Can you work these out from the model? Positions are in its coordinate system, mm. Face numbers are marked on the shaded views. A direction names the side the tool comes from. Coordinates: 2 decimals unless noted, no trailing zeros. Write each loop counter-clockwise with the first axis right and the second up, starting at its lowest first coordinate (ties: lowest second). Pieces come first, ordered by that corner, then holes. Notation, with made-up numbers: (-17.5, 48.5) - (16.5, 48.5) arc R6 ccw to (16.5, 53.5) - close; hole circle Ø11 at (38, 33.5). An arc over 180 degrees is marked (long way). One line per question, with ' | ' between items. Start each with the question number.
from build123d import *

# Parameters (mm, degrees)
SKETCH2_R           = 76.2
BOSS_EXTRUDE2_DEPTH = 50.8
FILLET1_R           = 25.4
SKETCH3_W           = 25.4
SKETCH3_H           = 25.4
BOSS_EXTRUDE3_DEPTH = 25.4
CUT_EXTRUDE2_REACH  = 154.532
SKETCH5_R           = 6.35
CUT_EXTRUDE3_REACH  = 154.532
SKETCH6_R           = 6.35


with BuildPart() as part:
    # Sketch2 → Boss-Extrude2 (new body)
    with BuildSketch(Plane(origin=(0, 0, 0), x_dir=(1, 0, 0), z_dir=(0, 1, 0))):
        with Locations(Location((0, 0, 0), (0, 0, 270))):
            Circle(SKETCH2_R)
    extrude(amount=BOSS_EXTRUDE2_DEPTH)

    # Fillet1
    fillet1_edges = [part.edges().sort_by_distance(p)[0] for p in [
        (0, 50.8, -76.2),
    ]]
    fillet(fillet1_edges, radius=FILLET1_R)

    # Sketch3 → Boss-Extrude3 (add)
    with BuildSketch(Plane(origin=(0, 50.8, 0), x_dir=(1, 0, 0), z_dir=(0, 1, 0))):
        with Locations((-19.05, 19.05)):
            Rectangle(SKETCH3_W, SKETCH3_H)
        with Locations((19.05, 19.05)):
            Rectangle(SKETCH3_W, SKETCH3_H)
        with Locations((-19.05, -19.05)):
            Rectangle(SKETCH3_W, SKETCH3_H)
        with Locations((19.05, -19.05)):
            Rectangle(SKETCH3_W, SKETCH3_H)
    extrude(amount=BOSS_EXTRUDE3_DEPTH)

    # Cut-Extrude2: up to this face of the body (flat: up to its plane)
    cut_extrude2_end = Plane(part.part.faces().sort_by_distance((31.75, 63.5, -19.05))[0])
    # Sketch5 → Cut-Extrude2 (cut, up to the picked face)
    with BuildSketch(Plane.ZY.offset(31.75), mode=Mode.PRIVATE) as cut_extrude2_sk1:
        with Locations((-19.05, 63.5)):
            Circle(SKETCH5_R)
    cut_extrude2_tool1 = split(extrude(cut_extrude2_sk1.sketch, amount=-CUT_EXTRUDE2_REACH, mode=Mode.PRIVATE), bisect_by=cut_extrude2_end, keep=Keep.BOTH, mode=Mode.PRIVATE)
    add(cut_extrude2_tool1.solids().sort_by(Axis((-31.75, 63.5, -19.05), (1, 0, 0)))[0], mode=Mode.SUBTRACT)

    # Cut-Extrude3: up to this face of the body (flat: up to its plane)
    cut_extrude3_end = Plane(part.part.faces().sort_by_distance((31.75, 63.5, 19.05))[0])
    # Sketch6 → Cut-Extrude3 (cut, up to the picked face)
    with BuildSketch(Plane.ZY.offset(31.75), mode=Mode.PRIVATE) as cut_extrude3_sk1:
        with Locations((19.05, 63.5)):
            Circle(SKETCH6_R)
    cut_extrude3_tool1 = split(extrude(cut_extrude3_sk1.sketch, amount=-CUT_EXTRUDE3_REACH, mode=Mode.PRIVATE), bisect_by=cut_extrude3_end, keep=Keep.BOTH, mode=Mode.PRIVATE)
    add(cut_extrude3_tool1.solids().sort_by(Axis((-31.75, 63.5, 19.05), (1, 0, 0)))[0], mode=Mode.SUBTRACT)


solid = part.part
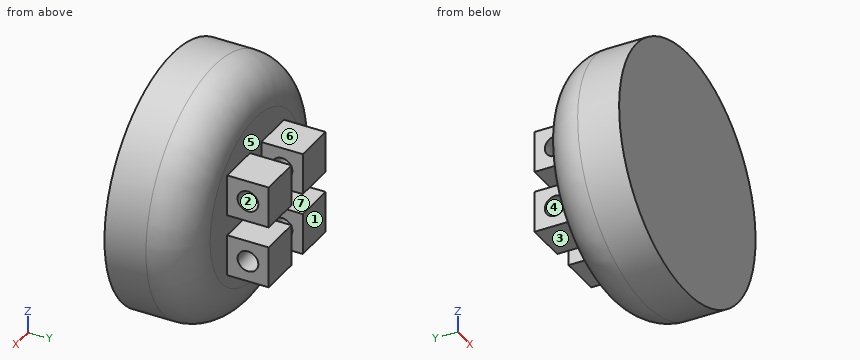
(1) If we section it at C-C on z = 0: List the corners of the cut face in (x, y) for me.
(2) If we mould it in two halves opening along Z, with no side actions, what happens to the marked faces 1, 2, 3 and 4? For each: +Z half, -Z half, draft (parallel to the pull), parting line (faces both ways), or undercut.
(3) If we section it at B-B on x = 0: List the corners of the cut face in (y, z) for me.
(4) Which directions (+Z, -Z, +X, -X, +Y, -Y) give clear straight access to the entire face, cutting with the end or side of a thin tool? Please do the marked faces 5, 6 and 7.
(5) If I drill on probe 1 along Z at (x, y) = (14, 63); probe 2 along Y at (x, z) = (-21.5, 19.05); probe 3 along X at (y, z) = (64.5, 9.5), over which ranges is the centre line in solid material (lowest first)?
(6) If we section it at A-A on y = 63.5: Give the number of separate pieces and of enclosed holes in the cut face, plus the area to 3 significant figures.
(7) I'm going to push flat-ended pins straight in: pin 1 (7.5 mm diameter, centred on x = 20.5, y = 65, fed in from +Z); pin 2 (20.5 mm diameter, centred on x = -24.5, y = 68, fed in from -Z); pin 3 (20.5 mm diameter, centred on x = -22.5, y = 58, fed in from -Z); pin 4 (10 mm diameter, centred on y = 63.5, z = 19.05, fed in from -X). Where does each tip first touch, or does it pass through?
Values:
1) outline: (-76.2, 0) - (76.2, 0) - (76.2, 25.4) arc R25.4 ccw to (50.8, 50.8) - (-50.8, 50.8) arc R25.4 ccw to (-76.2, 25.4) - close
2) face 1: draft | face 2: undercut | face 3: -Z half | face 4: undercut
3) outline: (0, -76.2) - (25.4, -76.2) arc R25.4 ccw to (50.8, -50.8) - (50.8, 50.8) arc R25.4 ccw to (25.4, 76.2) - (0, 76.2) - close
4) face 5: +Y | face 6: +Z, +X, -X, +Y | face 7: +X, -X, +Y
5) probe 1: -31.75 to -25.38, -12.72 to -6.35, 6.35 to 12.72, 25.38 to 31.75 | probe 2: 0 to 57.15, 69.85 to 76.2 | probe 3: -31.75 to -6.35, 6.35 to 31.75
6) separate pieces: 8 | enclosed holes: 0 | area: 1,290 mm2
7) pin 1: z = 31.75 | pin 2: z = -31.75 | pin 3: z = -59.05 | pin 4: through
